from build123d import *

# Parameters (mm, degrees)
ENL_V_MAT_EXTRU_1_DEPTH      = 1.5
R_P_TITION_CIRCULAIRE1_COUNT = 3


with BuildPart() as part:
    # Esquisse1 → R_volution1 (revolve)
    with BuildSketch(Plane.XY):
        with BuildLine():
            Line((-14, 4.86253393), (0, 4.86253393))
            Line((0, 4.86253393), (0, -16))
            add(Edge.make_bspline(
                [(-14, 4.86253393), (-12.085828485, -4.33132409), (-7.615170337, -16.338293634), (0, -16)],
                knots=[0, 0, 0, 0, 1, 1, 1, 1], degree=3))
        make_face()
    revolve(axis=Axis((0, 4.86253393, 0), (0, -1, 0)))

    # Esquisse2 → Enl_v. mat.-Extru.1 (cut, symmetric)
    with BuildSketch(Plane.XY):
        Polygon((13.219949482, 1.127759621), (8.325564148, 2.150008223), (7.712214987, -0.786622978), (12.60660032, -1.80887158), align=None)
    enl_v_mat_extru_1 = extrude(amount=ENL_V_MAT_EXTRU_1_DEPTH, both=True, mode=Mode.SUBTRACT)

    # R_p_tition circulaire1: Enl_v. mat.-Extru.1 ×3 about axis
    r_p_tition_circulaire1_axis = Axis((0, 0, 0), (0, 1, 0))
    for i in range(1, R_P_TITION_CIRCULAIRE1_COUNT):
        add(enl_v_mat_extru_1.rotate(r_p_tition_circulaire1_axis, i * 360 / R_P_TITION_CIRCULAIRE1_COUNT), mode=Mode.SUBTRACT)


solid = part.part
Verification items for the finished model (mm, model axes). Coordinates: 2 decimals unless noted, no trailing zeros. Answer as a JSON object with one key per item and string values. Group by question number.
Item 1: Scan lines: probe 1 along Z at (x, y) = (8.5, 0); probe 2 along Y at (x, z) = (-0.5, 9.75); probe 3 along X at (y, z) = (1, 9.75). Record each from-to range of solid material in increasing order.
Item 2: Depth check by flat-ended pin: pin 1 (3 mm diameter, centred on y = -13.5, z = -8, fed in from +X); pin 2 (1 mm diameter, centred on x = -2.5, y = -1.5, fed in from -Z); pin 3 (3 mm diameter, centred on x = -4.5, y = -5.5, fed in from -Z); pin 4 (4.5 mm diameter, centred on x = 9, y = -0.5, fed in from -Z). Enter the tip coordinate at first touch or a pass-through.
Item 3: Mould release check, pull along X, two halves, no side actions. Record for faces 1 (the flat face through (-5.37, 1.64, -9.34)), 2 (the flat face through (-5.4, 1.64, 9.32)), 3 (the flat face through (9.97, -1.26, 0.02)), 4 (the flat face through (0, 4.863, 0)): +X half, -X half, draft (parallel to the pull), parting line (faces both ways), or undercut.
Evaluation:
{
 "1": {"probe 1": "z = -9.57 to -1.5, 1.5 to 9.57", "probe 2": "y = -7.97 to 4.86", "probe 3": "x = -8.72 to -7.36, -3.9 to 8.72"},
 "2": {"pin 1": "passes through", "pin 2": "stops at z = -12.28", "pin 3": "stops at z = -10.79", "pin 4": "stops at z = -10.89"},
 "3": {"face 1": "undercut", "face 2": "undercut", "face 3": "+X half", "face 4": "draft"}
}
